```python
from build123d import *

# Parameters (mm, degrees)
F1_DEPTH = 24.892
F3_R     = 1.9249928247
F4_DEPTH = 25.4
F8_DEPTH = 25.4
F6_R     = 2.33692874
F9_DEPTH = 25.4
F10_R    = 5.08


with BuildPart() as f1:
    # F0 (on Front) → F1 (new body)
    with BuildSketch(Plane.XZ):
        with BuildLine():
            Line((-42.1696156263, 7.4068200774), (50.741981715, 7.4068200774))
            Line((50.741981715, 7.4068200774), (50.7852658629, 10.1576624438))
            Line((50.7852658629, 10.1576624438), (-42.5401590765, 10.1576624438))
            ThreePointArc((-42.5401590765, 10.1576624438), (-44.6625185823, 11.3214684612), (-44.2773737299, 13.7111374259))
            Line((-44.2773737299, 13.7111374259), (-27.9987339674, 30.3550571651))
            Line((-27.9987339674, 30.3550571651), (-29.7558531165, 32.0736132562))
            Line((-29.7558531165, 32.0736132562), (-46.0104458034, 15.4542801902))
            ThreePointArc((-46.0104458034, 15.4542801902), (-46.6281352998, 10.2191830011), (-42.1696156263, 7.4068200774))
        make_face()
    extrude(amount=F1_DEPTH)

    # F3 (on offset) → F4 (cut)
    with BuildSketch(Plane(origin=(-35.0542101214, 0, 34.2848840697), x_dir=(0, -1, 0), z_dir=(-0.7149082188, 0, 0.6992183055))):
        with Locations((4.9738232046, -6.1299321242)):
            Circle(F3_R)
        with Locations((18.6898232046, -6.1299321242)):
            Circle(F3_R)
    extrude(amount=-F4_DEPTH, mode=Mode.SUBTRACT)

    # F7 (on offset) → F8 (cut)
    with BuildSketch(Plane.XY.offset(17.78)):
        with BuildLine():
            ThreePointArc((9.39899395, -9.7591195918), (10.9418290691, -10.4711006155), (11.5712740591, -12.0494086295))
            ThreePointArc((11.5712740591, -12.0494086295), (11.0668007338, -13.4845114856), (9.7753070295, -14.2882885411))
            Line((9.7753070295, -14.2882885411), (33.0347828567, -14.2882885411))
            ThreePointArc((33.0347828567, -14.2882885411), (30.770198382, -12.0237040665), (33.0347828567, -9.7591195918))
            Line((33.0347828567, -9.7591195918), (9.39899395, -9.7591195918))
        make_face()
        with BuildLine():
            Line((33.0347828567, -14.2882885411), (33.0347828567, -9.7591195918))
            ThreePointArc((33.0347828567, -9.7591195918), (30.770198382, -12.0237040665), (33.0347828567, -14.2882885411))
        make_face()
        with BuildLine():
            ThreePointArc((35.2993673314, -12.0237040665), (34.6360858953, -10.4224010279), (33.0347828567, -9.7591195918))
            Line((33.0347828567, -9.7591195918), (33.0347828567, -14.2882885411))
            ThreePointArc((33.0347828567, -14.2882885411), (34.6360858953, -13.6250071051), (35.2993673314, -12.0237040665))
        make_face()
        with BuildLine():
            ThreePointArc((9.1565652679, -9.7591195918), (7.0053919382, -12.3598455256), (9.7753070295, -14.2882885411))
            Line((9.7753070295, -14.2882885411), (9.1565652679, -14.2882885411))
            Line((9.1565652679, -14.2882885411), (9.1565652679, -9.7591195918))
        make_face()
        with BuildLine():
            ThreePointArc((9.7753070295, -14.2882885411), (11.0668007338, -13.4845114856), (11.5712740591, -12.0494086295))
            ThreePointArc((11.5712740591, -12.0494086295), (10.9418290691, -10.4711006155), (9.39899395, -9.7591195918))
            Line((9.39899395, -9.7591195918), (9.1565652679, -9.7591195918))
            Line((9.1565652679, -9.7591195918), (9.1565652679, -14.2882885411))
            Line((9.1565652679, -14.2882885411), (9.7753070295, -14.2882885411))
        make_face()
    extrude(amount=-F8_DEPTH, mode=Mode.SUBTRACT)

    # F6 (on offset) → F9 (cut)
    with BuildSketch(Plane.XY.offset(17.78)):
        with Locations((-19.2057471722, -12.1737904847)):
            Circle(F6_R)
    extrude(amount=-F9_DEPTH, mode=Mode.SUBTRACT)

    # F10
    f10_edges = [f1.edges().sort_by_distance(p)[0] for p in [
        (-28.877294, 0, 31.214335),
        (-28.877294, -24.892, 31.214335),
        (50.763624, -24.892, 8.782241),
        (50.763624, 0, 8.782241),
    ]]
    fillet(f10_edges, radius=F10_R)


solid = f1.part
```
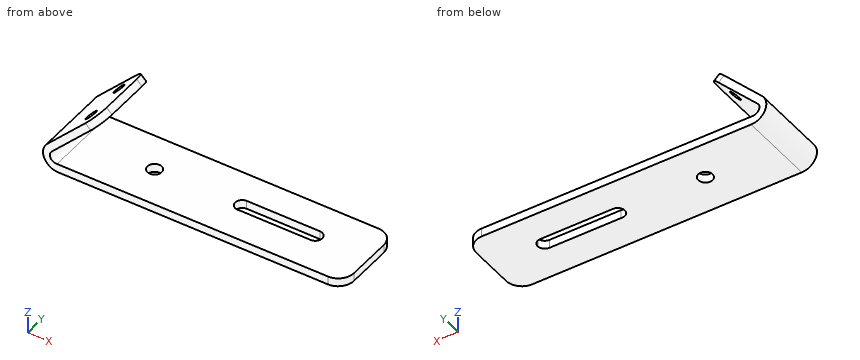
Verification items for the finished model (mm, model axes). Round coordinates to 2 decimals unless told otherwise and drop trailing zeros. Order: outer loops, then holes, each group sorted by start corner. A loop starts at its lowest first (then second) coordinate and runs counter-clockwise, first axis right, second up. Notation, with made-up numbers: (-38.5, 33) - (-21.5, 33) arc R17 cw to (-21.5, 60) - close; hole circle Ø5 at (65, 6). An arc over 180 degrees is marked (long way). Use CSV: the item, a comma, the result in double quotes. Start each with the question number.
1) Section check D-D, the plane z = 11.5. Record the cut outline in (x, y).
2) Thickness scan on L1, parallel to Z at x = 40, y = -23.5; L2, parallel to X at y = -3.25, z = 14.5; L3, parallel to X at y = -19.5, z = 17.25. Record the ranges inside material, lowest first.
3) Section check A-A, the plane x = 16. Record the cut outline in (y, z).
4) Go/stop test with flat-tipped pins: P1, Ø5, axis at y = -17.5, z = 20, coming from the +X side; P2, Ø10, axis at y = -6.5, z = 25.5, coming from the +X side; P3, Ø4, axis at x = -19.5, y = -21, coming from the +Z side. Record where each tip stops, or that it passes through.
5) Section check C-C, the plane y = -8.75. Record the cut outline in (x, z).
6) Section check B-B, the plane y = -18.5. Record the cut outline in (x, z), plus the area to 3 significant figures.
Answers:
1,outline,"(-47.04, -24.89) - (-44.74, -24.89) - (-44.74, 0) - (-47.04, 0) - close"
2,L1,"z = 7.41 to 10.16"
2,L2,"x = -46.62 to -43.51"
2,L3,"x = -44.25 to -40.82"
3,outline,"(-24.89, 7.41) - (-14.29, 7.41) - (-14.29, 10.16) - (-24.89, 10.16) - close; (-9.76, 7.41) - (0, 7.41) - (0, 10.16) - (-9.76, 10.16) - close"
4,P1,"stops at x = -35.68"
4,P2,"stops at x = -28"
4,P3,"stops at z = 10.16"
5,outline,"(-46.01, 15.45) arc R4.94 ccw to (-42.17, 7.41) - (50.74, 7.41) - (50.79, 10.16) - (-42.54, 10.16) arc R2.1 cw to (-44.28, 13.71) - (-28, 30.36) - (-29.76, 32.07) - close"
6,outline,"(-46.01, 15.45) arc R4.94 ccw to (-42.17, 7.41) - (50.74, 7.41) - (50.79, 10.16) - (-42.54, 10.16) arc R2.1 cw to (-44.28, 13.71) - (-35.11, 23.08) - (-36.87, 24.8) - close; (-34.19, 27.54) - (-32.43, 25.82) - (-28, 30.36) - (-29.76, 32.07) - close"
6,area,"323 mm²"
